from build123d import *

# Parameters (mm, degrees)
SKETCH_1_W          = 25
SKETCH_1_H          = 4
EXTRUDE_1_DEPTH     = 18
FILLET_1_R          = 1
SKETCH_3_R          = 1.6
CUT_EXTRUDE_2_DEPTH = 23.27666941
CUT_EXTRUDE_3_DEPTH = 2
CHAMFER_2_SIZE      = 3.5
CHAMFER_3_SIZE      = 3.5


with BuildPart() as part:
    # 草图1 → 凸台-拉伸1 (new body)
    with BuildSketch(Plane.XY):
        Rectangle(SKETCH_1_W, SKETCH_1_H)
    extrude(amount=EXTRUDE_1_DEPTH)

    # 圆角1
    fillet_1_edges = [part.edges().sort_by_distance(p)[0] for p in [
        (-12.5, 2, 9),
        (12.5, 2, 9),
        (12.5, -2, 9),
        (-12.5, -2, 9),
    ]]
    fillet(fillet_1_edges, radius=FILLET_1_R)

    # 草图3 → 切除-拉伸2 (cut, through all)
    with BuildSketch(Plane.XZ.offset(2)):
        with Locations((-7.5, 14)):
            Circle(SKETCH_3_R)
        with Locations((-7.5, 4)):
            Circle(SKETCH_3_R)
        with Locations(Location((7.5, 4, 0), (0, 0, 180))):
            Circle(SKETCH_3_R)
        with Locations(Location((7.5, 14, 0), (0, 0, 180))):
            Circle(SKETCH_3_R)
    extrude(amount=-CUT_EXTRUDE_2_DEPTH, mode=Mode.SUBTRACT)

    # 草图4 → 切除-拉伸3 (cut)
    with BuildSketch(Plane(origin=(0, 2, 0), x_dir=(1, 0, 0), z_dir=(0, 1, 0))):
        Polygon((5.570878435, 0), (3, -18), (-5.570878435, -18), (-3, 0), align=None)
    extrude(amount=-CUT_EXTRUDE_3_DEPTH, mode=Mode.SUBTRACT)

    # 倒角2
    # the kernel refuses this chamfer: 3.5 mm, written as the material it adds along each edge
    with BuildSketch(Plane(origin=(6.843529685, 0, -8.910465074), x_dir=(0.027219645584784704, 0.9996219169112968, 0.00388768887943796), z_dir=(-0.14139170518175465, 0, 0.9899537290731298))) as chamfer_2_piece_1_section:
        Polygon((CHAMFER_2_SIZE * 0.999621916911, CHAMFER_2_SIZE * 0.0274958766106), (-CHAMFER_2_SIZE * 0.0274958766106, CHAMFER_2_SIZE * 0.999621916911), (0, 0), align=None)
    chamfer_2_piece_1 = extrude(amount=36.184448925, mode=Mode.PRIVATE)
    chamfer_2_piece_1 = split(chamfer_2_piece_1, bisect_by=Plane(origin=(2.941803391, 0.818076093, 0), z_dir=(0, 0, 1)), keep=Keep.TOP, mode=Mode.PRIVATE)
    chamfer_2_piece_1 = split(chamfer_2_piece_1, bisect_by=Plane(origin=(2.941803391, 0.818076093, 18), z_dir=(0, 0, -1)), keep=Keep.TOP, mode=Mode.PRIVATE)
    chamfer_2_piece_1 = split(chamfer_2_piece_1, bisect_by=Plane(origin=(2.941803391, 2, 9), z_dir=(0, -1, 0)), keep=Keep.TOP, mode=Mode.PRIVATE)
    add(chamfer_2_piece_1)

    # 倒角3
    # the kernel refuses this chamfer: 3.5 mm, written as the material it adds along each edge
    with BuildSketch(Plane(origin=(-6.843529685, 0, 26.910465074), x_dir=(-0.02721964558478464, 0.9996219169112968, -0.003887688879437917), z_dir=(0.14139170518175467, 0, -0.9899537290731298))) as chamfer_3_piece_1_section:
        Polygon((CHAMFER_3_SIZE * 0.999621916911, CHAMFER_3_SIZE * 0.0274958766106), (-CHAMFER_3_SIZE * 0.0274958766106, CHAMFER_3_SIZE * 0.999621916911), (0, 0), align=None)
    chamfer_3_piece_1 = extrude(amount=36.184448925, mode=Mode.PRIVATE)
    chamfer_3_piece_1 = split(chamfer_3_piece_1, bisect_by=Plane(origin=(-2.941803391, 2, 9), z_dir=(0, -1, 0)), keep=Keep.TOP, mode=Mode.PRIVATE)
    chamfer_3_piece_1 = split(chamfer_3_piece_1, bisect_by=Plane(origin=(-2.941803391, 0.818076093, 18), z_dir=(0, 0, -1)), keep=Keep.TOP, mode=Mode.PRIVATE)
    chamfer_3_piece_1 = split(chamfer_3_piece_1, bisect_by=Plane(origin=(-2.941803391, 0.818076093, 0), z_dir=(0, 0, 1)), keep=Keep.TOP, mode=Mode.PRIVATE)
    add(chamfer_3_piece_1)


solid = part.part
Check sheet for the modelled part. Datum: model origin and axes. Units: mm. Round coordinates to 2 decimals unless told otherwise and drop trailing zeros. Loops run counter-clockwise (first coordinate to the right, second up) from the corner with the lowest first, then second, coordinate; pieces in that order, holes last.
1. Mould release check, pull along Z, two halves, no side actions. Record for faces 1 (the flat face through (-12.5, 0, 9)), 2 (the flat face through (0, 0, 0)), 3 (the flat face through (0, 0, 9)): released by +Z, released by -Z, zero draft, split by the parting line, or undercut.
2. Sectioned sample at C-C on z = 14. Record the boundary of the cut face in (x, y), and give its area (3 significant figures).
3. Sectioned sample at A-A on x = -7.5. Record the boundary of the cut face in (y, z).
4. Gauge pin test, flat end, axial feed: pin 1 Ø4.5 at (x, z) = (0, 10.5) entering from +Y. Record the tip position at first contact, or that the pin passes through.
5. Sectioned sample at D-D on y = -1.45. Record the boundary of the cut face in (x, z).
6. Sectioned sample at B-B on y = 0.6. Record the boundary of the cut face in (x, z).
7. Scan lines: probe 1 along Z at (x, y) = (-7.5, -0.9); probe 2 along X at (y, z) = (-1.7, 15.25); probe 3 along Z at (x, y) = (-8.5, -1.65). Record each from-to range of solid material in increasing order.
Recorded:
1. face 1: zero draft
1. face 2: released by -Z
1. face 3: undercut
2. outline: (-12.5, -1) arc R1 ccw to (-11.5, -2) - (-9.1, -2) - (-9.1, 2) - (-11.5, 2) arc R1 ccw to (-12.5, 1) - close; (-5.9, -2) - (5.9, -2) - (5.9, 2) - (2.06, 2) - (0.04, 0) - (-1.46, 0) - (-3.48, 2) - (-5.9, 2) - close; (9.1, -2) - (11.5, -2) arc R1 ccw to (12.5, -1) - (12.5, 1) arc R1 ccw to (11.5, 2) - (9.1, 2) - close
2. area: 66.5 mm2
3. outline: (-2, 0) - (2, 0) - (2, 2.4) - (-2, 2.4) - close; (-2, 5.6) - (2, 5.6) - (2, 12.4) - (-2, 12.4) - close; (-2, 15.6) - (2, 15.6) - (2, 18) - (-2, 18) - close
4. pin 1: stops at y = 1.72
5. outline: (-12.39, 0) - (12.39, 0) - (12.39, 18) - (-12.39, 18) - close; hole circle Ø3.2 at (-7.5, 4); hole circle Ø3.2 at (-7.5, 14); hole circle Ø3.2 at (7.5, 4); hole circle Ø3.2 at (7.5, 14)
6. outline: (-12.5, 0) - (-0.07, 0) - (-2.64, 18) - (-12.5, 18) - close; (0.07, 18) - (2.64, 0) - (12.5, 0) - (12.5, 18) - close; hole circle Ø3.2 at (-7.5, 4); hole circle Ø3.2 at (-7.5, 14); hole circle Ø3.2 at (7.5, 4); hole circle Ø3.2 at (7.5, 14)
7. probe 1: z = 0 to 2.4, 5.6 to 12.4, 15.6 to 18
7. probe 2: x = -12.21 to -8.5, -6.5 to 6.5, 8.5 to 12.21
7. probe 3: z = 0 to 2.75, 5.25 to 12.75, 15.25 to 18
